```python
from build123d import *

# Parameters (mm, degrees)
F1_DEPTH = 2
F2_R     = 4
F2_R_2   = 3.6
F3_DEPTH = 10
F4_R     = 2
F5_DEPTH = 10
F6_R     = 5.5
F6_R_2   = 4
F7_DEPTH = 0.5


with BuildPart() as f1:
    # F0 (on Front) → F1 (new body)
    with BuildSketch(Plane.XZ):
        with BuildLine():
            ThreePointArc((-10, 8.3066238629), (0, 13), (10, 8.3066238629))
            Line((10, 8.3066238629), (10, 25))
            Line((10, 25), (-10, 25))
            Line((-10, 25), (-10, 8.3066238629))
        make_face()
        with BuildLine():
            Line((10, 0), (10, 8.3066238629))
            ThreePointArc((10, 8.3066238629), (0, 13), (-10, 8.3066238629))
            Line((-10, 8.3066238629), (-10, 0))
            ThreePointArc((-10, 0), (0, 10), (10, 0))
        make_face()
        with BuildLine():
            Line((3.6, 0), (10, 0))
            ThreePointArc((10, 0), (0, 10), (-10, 0))
            Line((-10, 0), (-3.6, 0))
            ThreePointArc((-3.6, 0), (0, 3.6), (3.6, 0))
        make_face()
        with BuildLine():
            ThreePointArc((-10, 0), (0, -10), (10, 0))
            Line((10, 0), (3.6, 0))
            ThreePointArc((3.6, 0), (0, -3.6), (-3.6, 0))
            Line((-3.6, 0), (-10, 0))
        make_face()
    extrude(amount=F1_DEPTH)

    # F2 (on face) → F3 (join)
    with BuildSketch(Plane.XZ.offset(2)):
        Circle(F2_R)
        Circle(F2_R_2, mode=Mode.SUBTRACT)
    extrude(amount=F3_DEPTH)

    # F4 (on face) → F5 (join)
    with BuildSketch(Plane.XZ.offset(2)):
        with Locations((-6, 20)):
            Circle(F4_R)
        with Locations((6, 20)):
            Circle(F4_R)
    extrude(amount=F5_DEPTH)

    # F6 (on face) → F7 (join)
    with BuildSketch(Plane.XZ.offset(2)):
        Circle(F6_R)
        Circle(F6_R_2, mode=Mode.SUBTRACT)
    extrude(amount=F7_DEPTH)


solid = f1.part
```
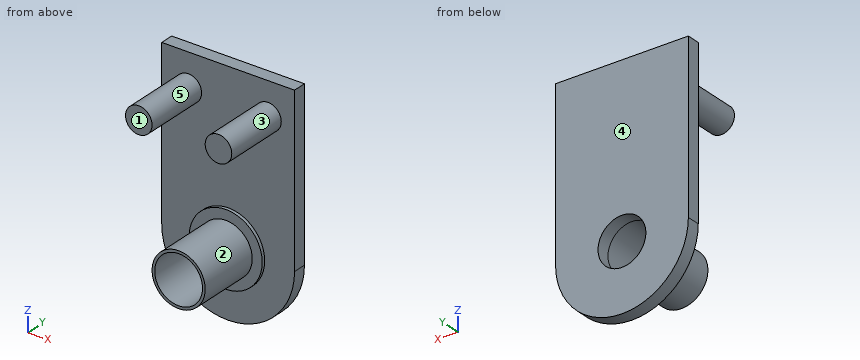
Part model, mm, in its own coordinate system. Face numbers are marked on the shaded views. A direction names the side the tool comes from. Round coordinates to 2 decimals unless told otherwise and drop trailing zeros. Loops run counter-clockwise (first coordinate to the right, second up) from the corner with the lowest first, then second, coordinate; pieces in that order, holes last.
Item 1: 3-axis set-ups, long thin cutter, end or side, ignore diameter. For the marked faces 4 and 5: which of +Z, -Z, +X, -X, +Y, -Y reach the whole face in a straight line?
Item 2: Cut at A-A, the plane x = 0. Give the cut face in (y, z).
Item 3: Drop flat-ended pins along their axis: P1, Ø3, axis at x = 3, z = 1.5, coming from the +Y side; P2, Ø2, axis at x = 0, z = 2.5, coming from the +Y side; P3, Ø1, axis at x = -6.5, z = 0, coming from the -Y side; P4, Ø3, axis at y = -10, z = 20, coming from the +X side. Give the stop position or say it passes through.
Item 4: Mould opens along X. For the marked faces 1, 2 and 3 say: +X half, -X half, draft (parallel to the pull), parting line (faces both ways), or undercut.
Item 5: Cut at B-B, the plane z = 20. Give the cut face in (x, y), then the cut area to 3 significant figures.
Item 6: Cut at D-D, the plane y = -11. Give the cut face in (x, z).
Item 7: Drill centre lines: line 1 (Z direction, x = 0, y = -5.75); line 2 (Y direction, x = -1.5, z = 22.5); line 3 (Y direction, x = 3, z = 4.5). Where is each one in solid material? Low to high.
Item 8: Cut at C-C, the plane y = -1.5. Give the cut face in (x, z).
A:
1. face 4: +Z, -Z, +X, -X, +Y
1. face 5: -Y
2. outline: (-12, -4) - (-2.5, -4) - (-2.5, -5.5) - (-2, -5.5) - (-2, -10) - (0, -10) - (0, -3.6) - (-12, -3.6) - close; (-12, 3.6) - (0, 3.6) - (0, 25) - (-2, 25) - (-2, 5.5) - (-2.5, 5.5) - (-2.5, 4) - (-12, 4) - close
3. P1: stops at y = 0
3. P2: passes through
3. P3: stops at y = -2
3. P4: stops at x = 8
4. face 1: draft
4. face 2: parting line
4. face 3: undercut
5. outline: (-10, -2) - (-8, -2) - (-8, -12) - (-4, -12) - (-4, -2) - (4, -2) - (4, -12) - (8, -12) - (8, -2) - (10, -2) - (10, 0) - (-10, 0) - close
5. area: 120 mm2
6. outline: circle Ø4 at (-6, 20); circle Ø8 at (0, 0); circle Ø4 at (6, 20); hole circle Ø7.2 at (0, 0)
7. line 1: z = -4 to -3.6, 3.6 to 4
7. line 2: y = -2 to 0
7. line 3: y = -2.5 to 0
8. outline: (-10, 0) arc R10 ccw to (10, 0) - (10, 25) - (-10, 25) - close; hole circle Ø7.2 at (0, 0)
